```python
from build123d import *

# Parameters (mm, degrees)
SKETCH1_R           = 27.5
SKETCH1_R_2         = 2
BOSS_EXTRUDE1_DEPTH = 18
CUT_EXTRUDE1_DEPTH  = 19
SKETCH3_R           = 15.675
CUT_EXTRUDE2_DEPTH  = 9.75
SKETCH5_R           = 3.75
CUT_EXTRUDE4_DEPTH  = 32.114098604


with BuildPart() as part:
    # Sketch1 → Boss-Extrude1 (new body)
    with BuildSketch(Plane.XY):
        Circle(SKETCH1_R)
        with Locations((0, 23.8125)):
            Circle(SKETCH1_R_2, mode=Mode.SUBTRACT)
        with Locations((20.622229928, 11.90625)):
            Circle(SKETCH1_R_2, mode=Mode.SUBTRACT)
        with Locations((20.622229928, -11.90625)):
            Circle(SKETCH1_R_2, mode=Mode.SUBTRACT)
        with Locations((0, -23.8125)):
            Circle(SKETCH1_R_2, mode=Mode.SUBTRACT)
        with Locations((-20.622229928, -11.90625)):
            Circle(SKETCH1_R_2, mode=Mode.SUBTRACT)
        with Locations((-20.622229928, 11.90625)):
            Circle(SKETCH1_R_2, mode=Mode.SUBTRACT)
    extrude(amount=BOSS_EXTRUDE1_DEPTH)

    # Sketch2 → Cut-Extrude1 (cut, through all)
    with BuildSketch(Plane(origin=(0, 0, 0), x_dir=(-1, 0, 0), z_dir=(0, 0, -1))):
        Polygon((0, 7.449665993), (-6.4516, 3.724832997), (-6.4516, -3.724832997), (0, -7.449665993), (6.4516, -3.724832997), (6.4516, 3.724832997), align=None)
    extrude(amount=-CUT_EXTRUDE1_DEPTH, mode=Mode.SUBTRACT)

    # Sketch3 → Cut-Extrude2 (cut)
    with BuildSketch(Plane(origin=(0, 0, 0), x_dir=(-1, 0, 0), z_dir=(0, 0, -1))):
        Circle(SKETCH3_R)
    extrude(amount=-CUT_EXTRUDE2_DEPTH, mode=Mode.SUBTRACT)

    # Sketch5 → Cut-Extrude4 (cut, through all)
    with BuildSketch(Plane(origin=(0.225707929, 7.31935346, 0), x_dir=(0.866025404, -0.5, 0), z_dir=(-0.5, -0.866025404, 0))):
        with Locations((-6.535792071, 4.426010426)):
            Circle(SKETCH5_R)
    extrude(amount=-CUT_EXTRUDE4_DEPTH, mode=Mode.SUBTRACT)


solid = part.part
```
The model under review builds one solid part; all positions refer to its coordinate system, in mm. A direction names the side the tool comes from. Coordinates: 2 decimals unless noted, no trailing zeros. Order: outer loops, then holes, each group sorted by start corner. A loop starts at its lowest first (then second) coordinate and runs counter-clockwise, first axis right, second up. Notation, with made-up numbers: (69, 50.25) -> (74, 50.25) arc R14 cw to (74, 57.25) -> close; hole circle Ø3 at (60, 17). An arc over 180 degrees is marked (long way). Answer in a Markdown table with one row per item. Add a question column.
Item 1: We need section A-A on y = 0. Write out the cut boundary in (x, z) (3 decimals).
Item 2: To check wall thickness, follow probe 1 along Y at (x, z) = (0, 9.5) (1 decimal); probe 2 along Y at (x, z) = (0, 5.75) (1 decimal); probe 3 along Y at (x, z) = (-22, 1.75). State the ranges of each line that lie inside material, in increasing order.
Item 3: We need section B-B on z = 3. Give the number of separate pieces and of enclosed holes in the cut face, plus the area to 3 significant figures.
Item 4: Mouldability with a two-part tool opening along Z and no side actions: class faces 4 (the flat face through (-3.2, -5.6, 13.8)), 5 (the flat face through (6, -6, 18)), 6 (the cylindrical face through (2.66, 20.58, 7.59)) as +Z half, -Z half, draft (parallel to the pull), parting line (faces both ways), or undercut.
Item 5: We need section C-C on x = 10.5. Write out the cut boundary in (y, z).
Item 6: Machinability: for faces 1 (the cylindrical face through (3.4, -15.3, 4.8)), 2 (the flat face through (3.27, -5.56, 13.82)), 3 (the flat face through (12, -12, 0)), which of the approach directions +Z, -Z, +X, -X, +Y, -Y give a long, thin tool a straight path to every point of the face, cutting with its end or side? Answer none if there is none.
Item 7: Clearance check with flat-ended pins moving along their axes: pin 1 (25 mm diameter, centred on x = -1.5, y = -6, fed in from -Z); pin 2 (2 mm diameter, centred on y = -14, z = 3, fed in from -X); pin 3 (3.5 mm diameter, centred on x = -20.62, y = 11.91, fed in from -Z); pin 4 (1 mm diameter, centred on x = 18.5, z = 4.5, fed in from -Y). State where each tip first meets the part, or that it passes through.
Final values:
| question | item | result |
|---|---|---|
| 1 | outline | (-27.5, 0) -> (-15.675, 0) -> (-15.675, 9.75) -> (-6.452, 9.75) -> (-6.452, 18) -> (-27.5, 18) -> close; (6.452, 9.75) -> (15.675, 9.75) -> (15.675, 0) -> (27.5, 0) -> (27.5, 18) -> (6.452, 18) -> close |
| 2 | probe 1 | y = -27.5 to -25.8, -21.8 to -15.7, 15.7 to 21.8, 25.8 to 27.5 |
| 2 | probe 2 | y = -27.5 to -25.8, -21.8 to -15.7, 27 to 27.5 |
| 2 | probe 3 | y = -16.5 to -13.36, -10.46 to 10.46, 13.36 to 16.5 |
| 3 | separate pieces | 1 |
| 3 | enclosed holes | 5 |
| 3 | area | 1,440 mm2 |
| 4 | face 4 | draft |
| 4 | face 5 | +Z half |
| 4 | face 6 | undercut |
| 5 | outline | (-25.42, 0) -> (-11.64, 0) -> (-11.64, 9.75) -> (11.64, 9.75) -> (11.64, 0) -> (25.42, 0) -> (25.42, 18) -> (-25.42, 18) -> close |
| 6 | face 1 | -Z |
| 6 | face 2 | +Z, -Z |
| 6 | face 3 | -Z, +X, -X, +Y, -Y |
| 7 | pin 1 | stops at z = 0 |
| 7 | pin 2 | stops at x = -24.23 |
| 7 | pin 3 | passes through |
| 7 | pin 4 | stops at y = -20.79 |
